Check sheet for the drawn part. Datum: minimum x, y, z corner. Units: mm. A direction names the side the tool comes from. Coordinates: 2 decimals unless noted, no trailing zeros. Loops run counter-clockwise (first coordinate to the right, second up) from the corner with the lowest first, then second, coordinate; pieces in that order, holes last.
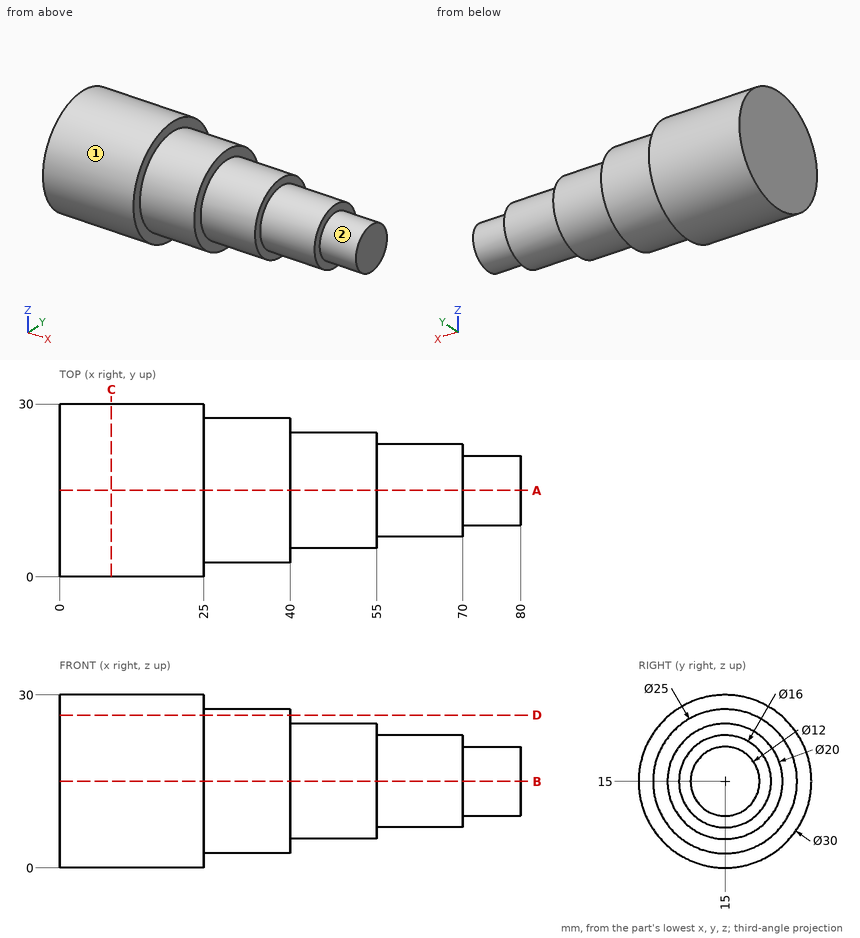
1) Set-up check for the marked faces 1 and 2: record each of +Z, -Z, +X, -X, +Y, -Y from which the full face is reachable in a straight line by a thin tool's end or side.
Answer sheet:
face 1: +X, -X
face 2: +X
2) Depth check by flat-ended pin: pin 1 (8 mm diameter, centred on x = 61, y = 11.5, fed in from -Z); pin 2 (12 mm diameter, centred on x = 42.5, z = 8.5, fed in from -Y); pin 3 (4 mm diameter, centred on x = 22, y = 7, fed in from -Z). Enter the tip coordinate at first touch or a pass-through.
Answer sheet:
pin 1: stops at z = 7
pin 2: stops at y = 2.54
pin 3: stops at z = 1.25
3) Section check A-A on y = 15. Enter the section's corners in (x, z), plus the area to 4 significant figures.
Answer sheet:
outline: (0, 0) - (25, 0) - (25, 2.5) - (40, 2.5) - (40, 5) - (55, 5) - (55, 7) - (70, 7) - (70, 9) - (80, 9) - (80, 21) - (70, 21) - (70, 23) - (55, 23) - (55, 25) - (40, 25) - (40, 27.5) - (25, 27.5) - (25, 30) - (0, 30) - close
area: 1,785 mm2
4) Scan lines: line 1 (X direction, y = 26.5, z = 16.5); line 2 (X direction, y = 2, z = 17.5); line 3 (Y direction, x = 54.5, z = 7). Record each from-to range of solid material in increasing order.
Answer sheet:
line 1: x = 0 to 40
line 2: x = 0 to 25
line 3: y = 9 to 21
5) Section check C-C on x = 9. Enter the section's corners in (y, z).
Answer sheet:
outline: circle Ø30 at (15, 15)
6) Section check D-D on z = 26.5. Enter the section's corners in (x, y).
Answer sheet:
outline: (0, 5.37) - (25, 5.37) - (25, 10.1) - (40, 10.1) - (40, 19.9) - (25, 19.9) - (25, 24.63) - (0, 24.63) - close
